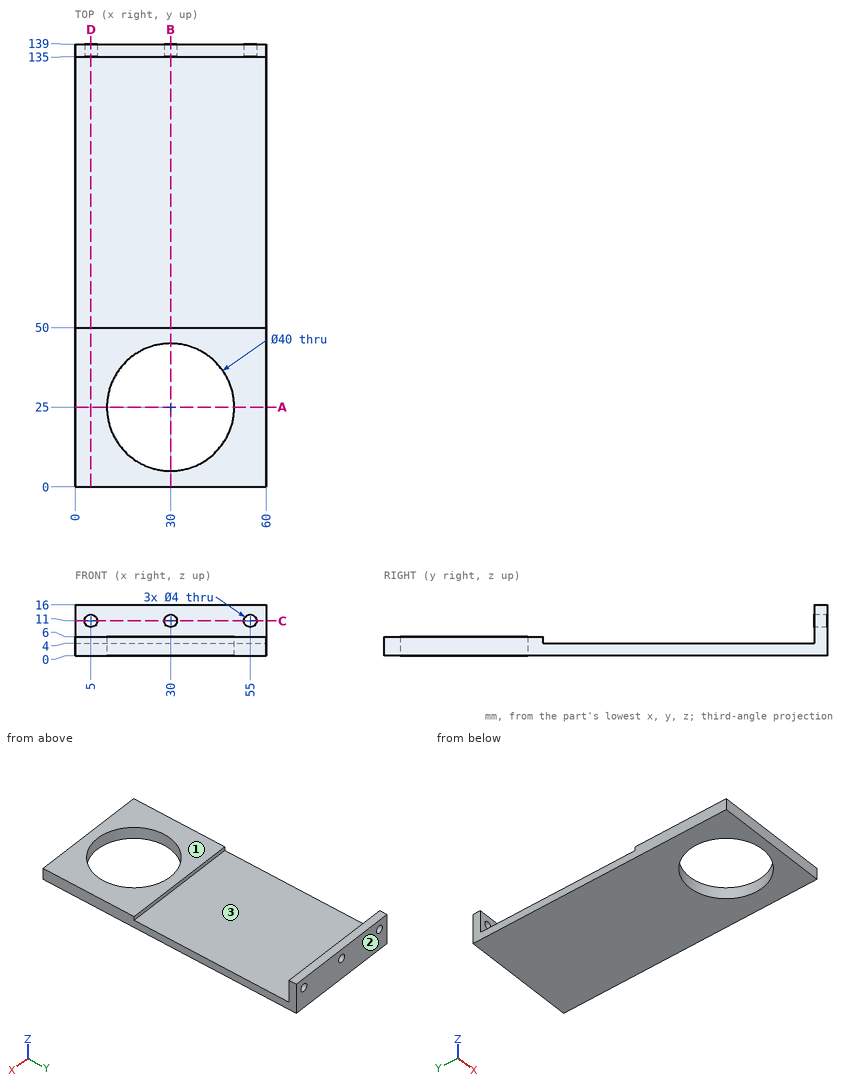
The figure shows three views and two pictorial views of one solid part (mm, origin at its lowest corner). Answer the questions. A direction names the side the tool comes from. Round coordinates to 2 decimals unless told otherwise and drop trailing zeros. Order: outer loops, then holes, each group sorted by start corner. A loop starts at its lowest first (then second) coordinate and runs counter-clockwise, first axis right, second up. Notation, with made-up numbers: M 72.5,62.5 L 80.5,62.5 A26 cw 80.5,101.5 Z; hole C -11,-33 d9. An arc over 180 degrees is marked long. Answer in a Markdown table with one row per item. Add a question column.
1) Flat-ended cylindrical pins translate along their axes: pin 1 Ø2.5 at (x, z) = (30, 11) entering from -Y; pin 2 Ø2 at (x, z) = (23, 8.5) entering from -Y; pin 3 Ø1 at (x, y) = (29.5, 98.5) entering from +Z. Find the tip coordinate at first contact, or state that the pin passes through.
2) Consider line 1 along X through (y, z) = (138.2, 11); line 2 along Y through (x, z) = (30.5, 1); line 3 along Y through (x, z) = (5.5, 5). Determine where each line is inside the solid, lowest interval first. Write a range as from..to.
3) The part is cut by section D-D on x = 5. Determine the outline of the cut face in (y, z), plus the area to 3 significant figures.
4) The part is cut by section B-B on x = 30. Determine the outline of the cut face in (y, z), plus the area to 3 significant figures.
5) Which of the six approach directions +Z, -Z, +X, -X, +Y, -Y give full straight-line access (tool end or side, diameter ignored) to the marked faces 1, 2 and 3?
6) The part is cut by section A-A on y = 25. Determine the outline of the cut face in (x, z).
7) The part is cut by section C-C on z = 11. Determine the outline of the cut face in (x, y), plus the area to 3 significant figures.
Findings below:
| question | item | result |
|---|---|---|
| 1 | pin 1 | passes through |
| 1 | pin 2 | stops at y = 135 |
| 1 | pin 3 | stops at z = 4 |
| 2 | line 1 | x = 0..3, 7..28, 32..53, 57..60 |
| 2 | line 2 | y = 0..5.01, 44.99..139 |
| 2 | line 3 | y = 0..50, 135..139 |
| 3 | outline | M 0,0 L 139,0 L 139,9 L 135,9 L 135,4 L 50,4 L 50,6 L 0,6 Z; M 135,13 L 139,13 L 139,16 L 135,16 Z |
| 3 | area | 688 mm² |
| 4 | outline | M 0,0 L 5,0 L 5,6 L 0,6 Z; M 45,0 L 139,0 L 139,9 L 135,9 L 135,4 L 50,4 L 50,6 L 45,6 Z; M 135,13 L 139,13 L 139,16 L 135,16 Z |
| 4 | area | 448 mm² |
| 5 | face 1 | +Z, +X, -X, -Y |
| 5 | face 2 | +Z, -Z, +X, -X, +Y |
| 5 | face 3 | +Z, +X, -X |
| 6 | outline | M 0,0 L 10,0 L 10,6 L 0,6 Z; M 50,0 L 60,0 L 60,6 L 50,6 Z |
| 7 | outline | M 0,135 L 3,135 L 3,139 L 0,139 Z; M 7,135 L 28,135 L 28,139 L 7,139 Z; M 32,135 L 53,135 L 53,139 L 32,139 Z; M 57,135 L 60,135 L 60,139 L 57,139 Z |
| 7 | area | 192 mm² |
